Check sheet for the drawn part. Datum: minimum x, y, z corner. Units: mm. A direction names the side the tool comes from. Round coordinates to 2 decimals unless told otherwise and drop trailing zeros. Write each loop counter-clockwise with the first axis right and the second up, starting at its lowest first coordinate (ties: lowest second). Pieces come first, ordered by that corner, then holes. Notation, with made-up numbers: (43.5, 20.25) -> (62.5, 20.25) arc R8 ccw to (62.5, 35.25) -> close; hole circle Ø5 at (12, 30.5). An arc over 180 degrees is marked (long way). Use a Markdown table: item, result.
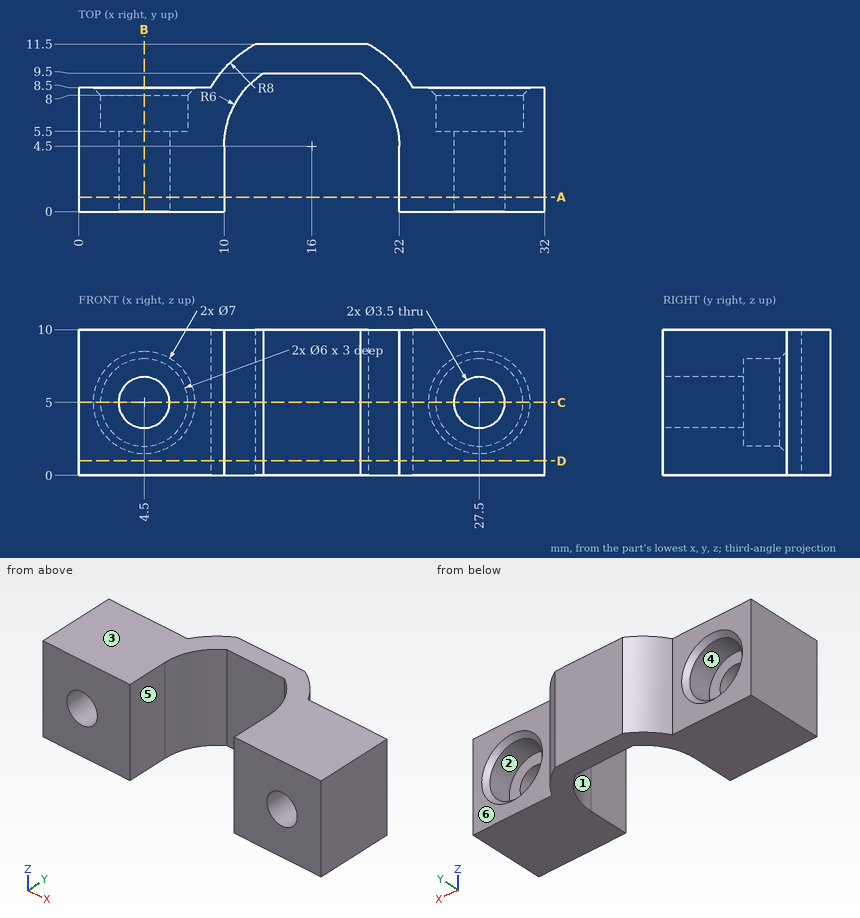
(1) Section check D-D on z = 1. Record the cut outline in (x, y).
A:
| item | result |
|---|---|
| outline | (0, 0) -> (10, 0) -> (10, 4.5) arc R6 cw to (12.68, 9.5) -> (19.32, 9.5) arc R6 cw to (22, 4.5) -> (22, 0) -> (32, 0) -> (32, 8.5) -> (22.93, 8.5) arc R8 ccw to (19.87, 11.5) -> (12.13, 11.5) arc R8 ccw to (9.07, 8.5) -> (0, 8.5) -> close |
(2) Access from +Z, -Z, +X, -X, +Y, -Y to the whole of each face (thin tool, end or side, straight path). Record for the marked faces 4, 5 and 6.
A:
| item | result |
|---|---|
| face 4 | +Y |
| face 5 | +Z, -Z, -Y |
| face 6 | +Z, -Z, +X, +Y |
(3) Release check for a two-part mould opening along Z. For the marked faces 1, 2 and 3 record: +Z half, -Z half, draft (parallel to the pull), parting line (faces both ways), or undercut.
A:
| item | result |
|---|---|
| face 1 | draft |
| face 2 | undercut |
| face 3 | +Z half |
(4) Section check A-A on y = 1. Record the cut outline in (x, z), plus the area to 3 significant figures.
A:
| item | result |
|---|---|
| outline | (0, 0) -> (10, 0) -> (10, 10) -> (0, 10) -> close; (22, 0) -> (32, 0) -> (32, 10) -> (22, 10) -> close; hole circle Ø3.5 at (4.5, 5); hole circle Ø3.5 at (27.5, 5) |
| area | 181 mm2 |
(5) Gauge pin test, flat ends, axial feed: pin 1 Ø4 at (y, z) = (2, 9) entering from -X; pin 2 Ø1 at (x, z) = (24, 6) entering from +Y; pin 3 Ø1.8 at (x, z) = (3.5, 5.5) entering from +Y; pin 4 Ø3 at (x, z) = (4.5, 5) entering from +Y. Record the tip position at first contact, or that the pin passes through.
A:
| item | result |
|---|---|
| pin 1 | stops at x = 0 |
| pin 2 | stops at y = 8.5 |
| pin 3 | stops at y = 5.5 |
| pin 4 | passes through |
(6) Section check C-C on z = 5. State how many separate pieces and enclosed holes the cut face has, plus the area to 3 significant figures.
A:
| item | result |
|---|---|
| separate pieces | 3 |
| enclosed holes | 0 |
| area | 125 mm2 |
(7) Thickness scan on line 1 (X direction, y = 2, z = 5); line 2 (Z direction, x = 27.5, y = 6.45); line 3 (Z direction, x = 4.5, y = 1.85). Record the ranges inside material, lowest first.
A:
| item | result |
|---|---|
| line 1 | x = 0 to 2.75, 6.25 to 10, 22 to 25.75, 29.25 to 32 |
| line 2 | z = 0 to 2, 8 to 10 |
| line 3 | z = 0 to 3.25, 6.75 to 10 |
(8) Section check B-B on x = 4.5. Record the cut outline in (y, z).
A:
| item | result |
|---|---|
| outline | (0, 0) -> (8.5, 0) -> (8.5, 1.5) -> (8, 2) -> (5.5, 2) -> (5.5, 3.25) -> (0, 3.25) -> close; (0, 6.75) -> (5.5, 6.75) -> (5.5, 8) -> (8, 8) -> (8.5, 8.5) -> (8.5, 10) -> (0, 10) -> close |
